```python
from build123d import *

# Parameters (mm, degrees)
CROQUIS1_W              = 20
CROQUIS1_H              = 12.7
SALIENTE_EXTRUIR1_DEPTH = 6.35


with BuildPart() as part:
    # Croquis1 → Saliente-Extruir1 (new, symmetric)
    with BuildSketch(Plane.XY):
        Rectangle(CROQUIS1_W, CROQUIS1_H)
    extrude(amount=SALIENTE_EXTRUIR1_DEPTH, both=True)

    # Croquis3 → Refrentado para tornillo con cabeza hueca de M61 (revolve, cut)
    with BuildSketch(Plane(origin=(0, 6.35, 0), x_dir=(0, 0, 1), z_dir=(1, 0, 0))):
        Polygon((0, 0), (0, 12.7), (3.325, 12.7), (3.3, 12.675), (3.3, 6.4), (5.5, 6.4), (5.5, 0.025), (5.525, 0), align=None)
    revolve(axis=Axis((0, 12.7, 0), (0, -1, 0)), mode=Mode.SUBTRACT)


solid = part.part
```
Geometry check sheet. Reference: the model listing, model coordinates, mm. A direction names the side the tool comes from. Coordinates: 2 decimals unless noted, no trailing zeros. Loops run counter-clockwise (first coordinate to the right, second up) from the corner with the lowest first, then second, coordinate; pieces in that order, holes last.
Item 1: Release check for a two-part mould opening along X. For faces 3 (the face through (-2.23, -3.14, -2.43)), 4 (the face through (-2, -6.35, -3)), 5 (the face through (10, 0, 0)) record: released by +X, released by -X, zero draft, split by the parting line, or undercut.
Item 2: Access from +Z, -Z, +X, -X, +Y, -Y to the whole of each face (thin tool, end or side, straight path). Record for faces 1 (the face through (0, -0.05, -4)), 2 (the face through (0, 6.35, -6)).
Item 3: Sectioned sample at A-A, the plane z = 0. Record the boundary of the cut face in (x, y) (3 decimals).
Item 4: Sectioned sample at B-B, the plane x = 0. Record the boundary of the cut face in (y, z) (3 decimals), then the cut area to 3 significant figures.
Item 5: Thickness scan on line 1 (X direction, y = 5, z = 0); line 2 (Z direction, x = 0, y = 2.25); line 3 (Z direction, x = 0, y = -3.5). Record the ranges inside material, lowest first.
Item 6: Go/stop test with a flat-tipped pin: pin 1 Ø2 at (x, z) = (-0.5, -0.5) entering from -Y. Record where the tip stops, or that it passes through.
Item 7: Sectioned sample at C-C, the plane y = -2.75. Record the boundary of the cut face in (x, z), then the cut area to 3 significant figures.
Check result:
1. face 3: undercut
1. face 4: zero draft
1. face 5: released by +X
2. face 1: +Y
2. face 2: +Z, -Z, +X, -X, +Y
3. outline: (-10, -6.35) - (-3.325, -6.35) - (-3.3, -6.325) - (-3.3, -0.05) - (-5.5, -0.05) - (-5.5, 6.325) - (-5.525, 6.35) - (-10, 6.35) - close; (3.3, -6.325) - (3.325, -6.35) - (10, -6.35) - (10, 6.35) - (5.525, 6.35) - (5.5, 6.325) - (5.5, -0.05) - (3.3, -0.05) - close
4. outline: (-6.35, -6.35) - (6.35, -6.35) - (6.35, -5.525) - (6.325, -5.5) - (-0.05, -5.5) - (-0.05, -3.3) - (-6.325, -3.3) - (-6.35, -3.325) - close; (-6.35, 3.325) - (-6.325, 3.3) - (-0.05, 3.3) - (-0.05, 5.5) - (6.325, 5.5) - (6.35, 5.525) - (6.35, 6.35) - (-6.35, 6.35) - close
4. area: 49.3 mm2
5. line 1: x = -10 to -5.5, 5.5 to 10
5. line 2: z = -6.35 to -5.5, 5.5 to 6.35
5. line 3: z = -6.35 to -3.3, 3.3 to 6.35
6. pin 1: passes through
7. outline: (-10, -6.35) - (10, -6.35) - (10, 6.35) - (-10, 6.35) - close; hole circle Ø6.6 at (0, 0)
7. area: 220 mm2
